Geometry: see drawing. Coordinates: mm, zero at the bounding-box minimum. A direction names the side the tool comes from. Coordinates: 2 decimals unless noted, no trailing zeros. Loops run counter-clockwise (first coordinate to the right, second up) from the corner with the lowest first, then second, coordinate; pieces in that order, holes last. Notation, with made-up numbers: (-22.75, 7.5) -> (-17.75, 7.5) arc R20 cw to (-17.75, 12.5) -> close; hole circle Ø7 at (50.25, -19.75). An arc over 180 degrees is marked (long way). One line per question, with ' | ' between items. Start each with the question number.
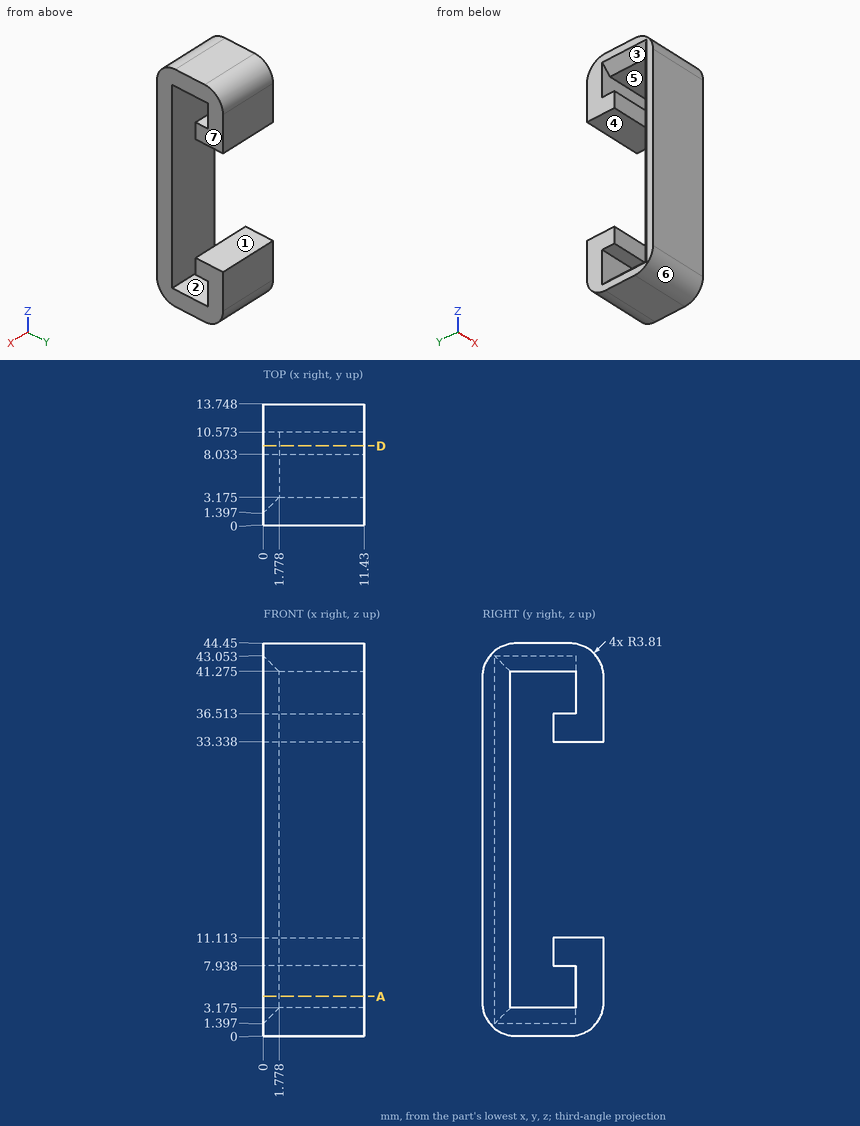
(1) Contact query for flat-ended pins moving along their axis: pin 1 Ø5 at (y, z) = (6, 21.5) entering from +X; pin 2 Ø3 at (x, z) = (6, 30.5) entering from +Y (1 decimal). Output: stop coordinate, or through.
(2) Draft query along Z for the marked faces 4, 5, 6 and 7. Return one class per face: pulls with the +Z half, pulls with the -Z half, needs draft (parallel to the pull), parting line crosses it, or undercut.
(3) Cut plane A-A, the plane z = 4.5. Return the cut outline in (x, y) (1 decimal).
(4) Cut plane D-D, the plane y = 9. State how many separate pieces and enclosed holes the cut face has, and give its area (3 significant figures).
(5) Access query for the marked faces 1, 2 and 3. Directions: +Z, -Z, +X, -X, +Y, -Y. A direction counts if a zero-diameter tool reaches every point of the face in a straight line with its end or side. Return the directions, or none.
(6) Ray query, L1, parallel to Y at x = 10, z = 40.5 (1 decimal); L2, parallel to Y at x = 2.75, z = 11 (1 decimal); L3, parallel to Y at x = 5.5, z = 30.5 (1 decimal). Return the intervals inside material, ascending.
Here are the results:
1) pin 1: passes through | pin 2: stops at y = 3.2
2) face 4: undercut | face 5: undercut | face 6: pulls with the -Z half | face 7: needs draft
3) outline: (0, 0) -> (11.4, 0) -> (11.4, 3.2) -> (1.8, 3.2) -> (0, 1.4) -> close; (0, 10.6) -> (11.4, 10.6) -> (11.4, 13.7) -> (0, 13.7) -> close
4) separate pieces: 4 | enclosed holes: 0 | area: 142 mm2
5) face 1: +X, -X, +Y | face 2: +X, -X | face 3: -X
6) L1: y = 0 to 3.2, 10.6 to 13.7 | L2: y = 0 to 3.2, 8 to 13.7 | L3: y = 0 to 3.2
